from build123d import *

# Parameters (mm, degrees)
SKETCH1_R           = 2
BOSS_EXTRUDE1_DEPTH = 15
SKETCH2_R           = 2.25
CUT_EXTRUDE1_DEPTH  = 8
SKETCH3_R           = 3.75
CUT_EXTRUDE2_DEPTH  = 60.172282871
SKETCH4_W           = 61.794010768
SKETCH4_H           = 5
CUT_EXTRUDE3_DEPTH  = 58.873647372


with BuildPart() as part:
    # Sketch1 → Boss-Extrude1 (new body)
    with BuildSketch(Plane(origin=(0, 0, 0), x_dir=(-1, 0, 0), z_dir=(0, 1, 0))):
        with BuildLine():
            Line((20.35, 10), (20.35, -10))
            Line((20.35, -10), (-20.35, -10))
            Line((-20.35, -10), (-20.35, 10))
            Line((-20.35, 10), (-30.35, 10))
            Line((-30.35, 10), (-30.35, -15.660254038))
            ThreePointArc((-30.35, -15.660254038), (-30.520370869, -16.954349263), (-31.019872981, -18.160254038))
            Line((-31.019872981, -18.160254038), (-41.897005384, -37))
            Line((-41.897005384, -37), (41.897005384, -37))
            Line((41.897005384, -37), (31.019872981, -18.160254038))
            ThreePointArc((31.019872981, -18.160254038), (30.520370869, -16.954349263), (30.35, -15.660254038))
            Line((30.35, -15.660254038), (30.35, 10))
            Line((30.35, 10), (20.35, 10))
        make_face()
        with Locations(Location((23.85, -5, 0), (0, 0, 90))):
            Circle(SKETCH1_R, mode=Mode.SUBTRACT)
        with Locations(Location((23.85, 5, 0), (0, 0, 90))):
            Circle(SKETCH1_R, mode=Mode.SUBTRACT)
        with Locations(Location((-23.85, -5, 0), (0, 0, 270))):
            Circle(SKETCH1_R, mode=Mode.SUBTRACT)
        with Locations(Location((-23.85, 5, 0), (0, 0, 270))):
            Circle(SKETCH1_R, mode=Mode.SUBTRACT)
    extrude(amount=-BOSS_EXTRUDE1_DEPTH)

    # Sketch2 → Cut-Extrude1 (cut)
    with BuildSketch(Plane(origin=(0, 0, -37), x_dir=(1, 0, 0), z_dir=(0, 0, -1))):
        with Locations(Location((-34.897005384, 7.5, 0), (0, 0, 180))):
            Circle(SKETCH2_R)
        with Locations((34.897005384, 7.5)):
            Circle(SKETCH2_R)
    extrude(amount=-CUT_EXTRUDE1_DEPTH, mode=Mode.SUBTRACT)

    # Sketch3 → Cut-Extrude2 (cut, through all)
    with BuildSketch(Plane(origin=(0, 0, -29), x_dir=(-1, 0, 0), z_dir=(0, 0, -1))):
        with Locations((-34.897005384, -7.5)):
            Circle(SKETCH3_R)
        with Locations((34.897005384, -7.5)):
            Circle(SKETCH3_R)
    extrude(amount=-CUT_EXTRUDE2_DEPTH, mode=Mode.SUBTRACT)

    # Sketch4 → Cut-Extrude3 (cut, through all)
    with BuildSketch(Plane.XZ.offset(15)):
        with Locations((0, -34.5)):
            Rectangle(SKETCH4_W, SKETCH4_H)
    extrude(amount=-CUT_EXTRUDE3_DEPTH, mode=Mode.SUBTRACT)


solid = part.part
Input: part model. Units: mm. Frame: model coordinates. A direction names the side the tool comes from. Round coordinates to 2 decimals unless told otherwise and drop trailing zeros. Write each loop counter-clockwise with the first axis right and the second up, starting at its lowest first coordinate (ties: lowest second). Pieces come first, ordered by that corner, then holes.
1) Draft query along Y for faces 1 (the flat face through (20.35, -7, 0)), 2 (the flat face through (1, 0, -18)), 3 (the cylindrical face through (-31.15, -7.38, -24.83)). Return one class per face: pulls with the +Y half, pulls with the -Y half, needs draft (parallel to the pull), parting line crosses it, or undercut.
2) Reachability of faces 4 (the flat face through (0, -7, -10)), 5 (the cylindrical face through (-21.867, -7.395, 4.74)), 6 (the flat face through (-32, -7, -29)), 7 (the flat face through (-37.743, -7.395, -29.805)), 8 (the flat face through (30.897, -8, -35)) from +Z, -Z, +X, -X, +Y, -Y: full face, straight path, thin tool, end or side. Return the list, or none.
3) Ray query, L1, parallel to Z at x = -24, y = -0.75; L2, parallel to X at y = -6, z = -5; L3, parallel to X at y = -6, z = -7.5. Return the intervals inside material, ascending.
4) Cut plane A-A (y = -7.5). Count the separate pieces of the cut face and the enclosed holes in it, then the cut area to 3 significant figures.
5) Cut plane C-C (y = -1). Return the cut outline in (x, z).
6) Contact query for flat-ended pins moving along their axis: P1, Ø4.5, axis at y = -7, z = -3.5, coming from the -X side; P2, Ø3, axis at x = 34, y = -8, coming from the +Z side; P3, Ø4, axis at y = -8, z = -28.5, coming from the -X side. Output: stop coordinate, or through.
7) Cut plane D-D (z = -27.5). Return the cut outline in (x, y).
8) Cut plane B-B (z = 5). Return the cut outline in (x, y), then the cut area to 3 significant figures.
Geometry says:
1. face 1: needs draft
1. face 2: pulls with the +Y half
1. face 3: undercut
2. face 4: +Z, +Y, -Y
2. face 5: +Y, -Y
2. face 6: +Z
2. face 7: +Z, -X, +Y, -Y
2. face 8: -Z, +Y, -Y
3. L1: z = -32 to -6.99, -3.01 to 3.01, 6.99 to 10
3. L2: x = -30.35 to -25.85, -21.85 to -20.35, 20.35 to 21.85, 25.85 to 30.35
3. L3: x = -30.35 to -20.35, 20.35 to 30.35
4. separate pieces: 3
4. enclosed holes: 4
4. area: 1,770 mm2
5. outline: (-41.9, -37) - (-30.9, -37) - (-30.9, -32) - (30.9, -32) - (30.9, -37) - (41.9, -37) - (31.02, -18.16) arc R5 cw to (30.35, -15.66) - (30.35, 10) - (20.35, 10) - (20.35, -10) - (-20.35, -10) - (-20.35, 10) - (-30.35, 10) - (-30.35, -15.66) arc R5 cw to (-31.02, -18.16) - close; hole circle Ø4 at (-23.85, -5); hole circle Ø4 at (-23.85, 5); hole circle Ø4 at (23.85, -5); hole circle Ø4 at (23.85, 5)
6. P1: stops at x = -30.35
6. P2: stops at z = -29
6. P3: stops at x = -38.14
7. outline: (-36.41, -15) - (36.41, -15) - (36.41, -10.93) arc R3.75 cw (long way) to (36.41, -4.07) - (36.41, 0) - (-36.41, 0) - (-36.41, -4.07) arc R3.75 cw (long way) to (-36.41, -10.93) - close
8. outline: (-30.35, -15) - (-25.85, -15) - (-25.85, 0) - (-30.35, 0) - close; (-21.85, -15) - (-20.35, -15) - (-20.35, 0) - (-21.85, 0) - close; (20.35, -15) - (21.85, -15) - (21.85, 0) - (20.35, 0) - close; (25.85, -15) - (30.35, -15) - (30.35, 0) - (25.85, 0) - close
8. area: 180 mm2
